from build123d import *

# Parameters (mm, degrees)
BOSS_EXTRUDE1_DEPTH     = 2.54
SKETCH11_W              = 3.81
SKETCH11_H              = 11.43
SKETCH11_W_2            = 8.382
SKETCH11_H_2            = 8.382
CUT_EXTRUDE1_DEPTH      = 1
CUT_EXTRUDE1_DEPTH_BACK = 3.54
SKETCH12_R              = 1.27
CUT_EXTRUDE2_DEPTH      = 1
CUT_EXTRUDE2_DEPTH_BACK = 3.54
SKETCH13_R              = 1.27
CUT_EXTRUDE3_DEPTH      = 1
CUT_EXTRUDE3_DEPTH_BACK = 3.54
SKETCH14_W              = 3.556
SKETCH14_H              = 13.97
CUT_EXTRUDE4_DEPTH      = 1
CUT_EXTRUDE4_DEPTH_BACK = 3.54
SKETCH16_R              = 1.27
CUT_EXTRUDE5_DEPTH      = 1
CUT_EXTRUDE5_DEPTH_BACK = 3.54


with BuildPart() as part:
    # Sketch10 → Boss-Extrude1 (new body)
    with BuildSketch(Plane.XY):
        with BuildLine():
            Line((53.34, 1.27), (53.34, -92.71))
            ThreePointArc((53.34, -92.71), (51.852102448, -96.302102448), (48.26, -97.79))
            Line((48.26, -97.79), (16.846989059, -97.79))
            ThreePointArc((16.846989059, -97.79), (15.638688158, -97.644208035), (14.499741809, -97.215200367))
            Line((14.499741809, -97.215200367), (-16.7505185, -80.933552139))
            ThreePointArc((-16.7505185, -80.933552139), (-18.059258376, -79.955412607), (-18.989802686, -78.61241436))
            Line((-18.989802686, -78.61241436), (-28.309569459, -59.040904135))
            ThreePointArc((-28.309569459, -59.040904135), (-28.795802898, -57.127870198), (-28.51617555, -55.173917704))
            Line((-28.51617555, -55.173917704), (-8.107195629, 2.952923842))
            ThreePointArc((-8.107195629, 2.952923842), (-6.251501454, 5.414614163), (-3.314058103, 6.35))
            Line((-3.314058103, 6.35), (48.26, 6.35))
            ThreePointArc((48.26, 6.35), (51.852102448, 4.862102448), (53.34, 1.27))
        make_face()
    extrude(amount=BOSS_EXTRUDE1_DEPTH)

    # Sketch11 → Cut-Extrude1 (cut, two sides)
    with BuildSketch(Plane.XY.offset(2.54)) as cut_extrude1_sk:
        with Locations((31.65602, -79.121)):
            Rectangle(SKETCH11_W, SKETCH11_H)
        with Locations((23.78202, -79.121)):
            Rectangle(SKETCH11_W, SKETCH11_H)
        with Locations((3.878385852, -55.88)):
            Rectangle(SKETCH11_W_2, SKETCH11_H_2)
        with Locations((-5.011614148, -46.99)):
            Rectangle(SKETCH11_W_2, SKETCH11_H_2)
        with Locations((3.878385852, -38.1)):
            Rectangle(SKETCH11_W_2, SKETCH11_H_2)
        with Locations((12.768385852, -46.99)):
            Rectangle(SKETCH11_W_2, SKETCH11_H_2)
        with Locations((-9.017, -64.897)):
            Rectangle(SKETCH11_W_2, SKETCH11_H_2)
        with Locations((3.175, -70.485)):
            Rectangle(SKETCH11_W_2, SKETCH11_H_2)
        with Locations((15.367, -76.073)):
            Rectangle(SKETCH11_W_2, SKETCH11_H_2)
    extrude(amount=CUT_EXTRUDE1_DEPTH, mode=Mode.SUBTRACT)
    extrude(cut_extrude1_sk.sketch, amount=-CUT_EXTRUDE1_DEPTH_BACK, mode=Mode.SUBTRACT)

    # Sketch12 → Cut-Extrude2 (cut, two sides)
    with BuildSketch(Plane(origin=(0, 0, 0), x_dir=(-1, 0, 0), z_dir=(0, 0, -1))) as cut_extrude2_sk:
        with Locations((18.034, -57.15)):
            Circle(SKETCH12_R)
        with Locations((-43.942, -85.852)):
            Circle(SKETCH12_R)
    extrude(amount=CUT_EXTRUDE2_DEPTH, mode=Mode.SUBTRACT)
    extrude(cut_extrude2_sk.sketch, amount=-CUT_EXTRUDE2_DEPTH_BACK, mode=Mode.SUBTRACT)

    # Sketch13 → Cut-Extrude3 (cut, two sides)
    with BuildSketch(Plane(origin=(0, 0, 0), x_dir=(-1, 0, 0), z_dir=(0, 0, -1))) as cut_extrude3_sk:
        with Locations((25.012261453, -59.761967182)):
            Circle(SKETCH13_R)
        with Locations((-48.0822, 2.286)):
            Circle(SKETCH13_R)
        with Locations((3.718687848, 1.651)):
            Circle(SKETCH13_R)
    extrude(amount=CUT_EXTRUDE3_DEPTH, mode=Mode.SUBTRACT)
    extrude(cut_extrude3_sk.sketch, amount=-CUT_EXTRUDE3_DEPTH_BACK, mode=Mode.SUBTRACT)

    # Sketch14 → Cut-Extrude4 (cut, two sides)
    with BuildSketch(Plane(origin=(0, 0, 0), x_dir=(-1, 0, 0), z_dir=(0, 0, -1))) as cut_extrude4_sk:
        with Locations((-35.010498686, -19.798068862)):
            Rectangle(SKETCH14_W, SKETCH14_H)
    extrude(amount=CUT_EXTRUDE4_DEPTH, mode=Mode.SUBTRACT)
    extrude(cut_extrude4_sk.sketch, amount=-CUT_EXTRUDE4_DEPTH_BACK, mode=Mode.SUBTRACT)

    # Sketch16 → Cut-Extrude5 (cut, two sides)
    with BuildSketch(Plane(origin=(0, 0, 0), x_dir=(-1, 0, 0), z_dir=(0, 0, -1))) as cut_extrude5_sk:
        with Locations((-32.21898687, -9.676053038)):
            Circle(SKETCH16_R)
    extrude(amount=CUT_EXTRUDE5_DEPTH, mode=Mode.SUBTRACT)
    extrude(cut_extrude5_sk.sketch, amount=-CUT_EXTRUDE5_DEPTH_BACK, mode=Mode.SUBTRACT)


solid = part.part
Can you work these out from the model? Positions are in its coordinate system, mm. Give positions to 0.01 mm unless a question says otherwise; leave off trailing zeros. Loops run counter-clockwise (first coordinate to the right, second up) from the corner with the lowest first, then second, coordinate; pieces in that order, holes last. Notation, with made-up numbers: (26.25, 25) -> (52.25, 25) arc R16 cw to (52.25, 36) -> close; hole circle Ø10 at (66.25, 0.5). An arc over 180 degrees is marked (long way). Write item = value, one per line.
1) Suppose I cut it at D-D on y = -30. Write out the boundary of the cut face in (x, z).
Check result:
outline = (-19.68, 0) -> (53.34, 0) -> (53.34, 2.54) -> (-19.68, 2.54) -> close
2) Suppose I cut it at A-A on y = -41. Write out the boundary of the cut face in (x, z).
Check result:
outline = (-23.54, 0) -> (-0.31, 0) -> (-0.31, 2.54) -> (-23.54, 2.54) -> close; (8.07, 0) -> (53.34, 0) -> (53.34, 2.54) -> (8.07, 2.54) -> close
3) Will this pin go through, and if not, where does the flat tip stop? pin 1 (0.8 mm diameter, centred on y = -80.5, z = 1, fed in from -X).
Check result:
pin_1 = -17.91
4) Thinking about a two-plate mould opening in Y: for faces 1 (the cylindrical face through (-18.043, -79.972, 1.252)), 2 (the flat face through (4, -60.071, 1)), 3 (the cylindrical face through (51.812, 4.901, 1.252)), which applies, released by +Y, released by -Y, zero draft, split by the parting line, or undercut?
Check result:
face_1 = released by -Y
face_2 = undercut
face_3 = released by +Y
5) I need wall thicknesses on L1, parallel to Y at x = 14.5, z = 0.85; L2, parallel to Y at x = 36, z = 1.5; L3, parallel to Y at x = 17, z = 1.1. Which ranges of each line are inside material? Lowest first, please. Write a range as from..to.
Check result:
L1 = -97.22..-80.26, -71.88..-51.18, -42.8..6.35
L2 = -97.79..-26.78, -12.81..6.35
L3 = -97.79..-80.26, -71.88..6.35
6) Suppose I cut it at C-C on z = 1.3. Give the number of separate pieces and of enclosed holes in the cut face, then the cut area to 3 significant figures.
Check result:
separate_pieces = 1
enclosed_holes = 16
area = 6,600 mm2
7) Suppose I cut it at B-B on y = -57.15. Write out the boundary of the cut face in (x, z), then the cut area to 3 significant figures.
Check result:
outline = (-28.79, 0) -> (-19.3, 0) -> (-19.3, 2.54) -> (-28.79, 2.54) -> close; (-16.76, 0) -> (-0.31, 0) -> (-0.31, 2.54) -> (-16.76, 2.54) -> close; (8.07, 0) -> (53.34, 0) -> (53.34, 2.54) -> (8.07, 2.54) -> close
area = 181 mm2
